Source: CAD feature listing. Evaluate the final solid. Frame: model axes, mm. A direction names the side the tool comes from. Give positions to 0.01 mm unless a question says otherwise; leave off trailing zeros. Order: outer loops, then holes, each group sorted by start corner. A loop starts at its lowest first (then second) coordinate and runs counter-clockwise, first axis right, second up.
1) Section C-C, the plane x = -3.25. Return loops of the section in (y, z).
2) Material intervals for line 1 (Y direction, x = -5, z = 7.5); line 2 (Z direction, x = 9.5, y = -14.25); line 3 (Z direction, x = 7.5, y = -14.5), sorted ascending.
3) First-contact query: P1, Ø5, axis at x = 2.5, z = 6, coming from the +Y side; P2, Ø2, axis at x = 10, z = -1.5, coming from the -Y side. Flat tips, straight axial feed; report the tip coordinate or a pass-through.
4) Access query for faces 5 (the face through (0, -12.7, -4)), 6 (the face through (-8, -17.018, -12)). Directions: +Z, -Z, +X, -X, +Y, -Y. A direction counts if a zero-diameter tool reaches every point of the face in a straight line with its end or side. Return the directions, or none.
5) Section A-A, the plane x = 8.25. Return loops of the section in (y, z).
6) Draft query along X for faces 1 (the face through (-4.62, -14.83, 5.84)), 2 (the face through (-12.639, -6, -4)), 3 (the face through (12.761, -6, -4)), 4 (the face through (0, -6, -16.45)). Return one class per face: released by +X, released by -X, zero draft, split by the parting line, or undercut.
7) Section B-B, the plane z = 6.5. Return loops of the section in (x, y).
8) Section D-D, the plane z = -6.75. Return loops of the section in (x, y), plus the area to 3 significant figures.
```python
from build123d import *

# Parameters (mm, degrees)
F0_W     = 25.4
F0_H     = 25.4
F1_DEPTH = 12.7
F2_R     = 3.892272
F3_DEPTH = 17.018
F2_R_2   = 3.825823
F4_DEPTH = 17.018
F2_R_3   = 3.864432
F5_DEPTH = 17.018
F2_R_4   = 3.786819
F6_DEPTH = 17.018


with BuildPart() as f1:
    # F0 (on Front) → F1 (new body)
    with BuildSketch(Plane.XZ):
        with Locations((0.061012, -3.750413)):
            Rectangle(F0_W, F0_H)
    extrude(amount=F1_DEPTH)

    # F2 (on Front) → F3 (join)
    with BuildSketch(Plane.XZ):
        with Locations((-8.308703, -12.045457)):
            Circle(F2_R)
    extrude(amount=F3_DEPTH)

    # F2 (on Front) → F4 (join)
    with BuildSketch(Plane.XZ):
        with Locations((8.594656, -12.16163)):
            Circle(F2_R_2)
    extrude(amount=F4_DEPTH)

    # F2 (on Front) → F5 (join)
    with BuildSketch(Plane.XZ):
        with Locations((-8.308703, 4.683642)):
            Circle(F2_R_3)
    extrude(amount=F5_DEPTH)

    # F2 (on Front) → F6 (join)
    with BuildSketch(Plane.XZ):
        with Locations((8.594656, 4.683642)):
            Circle(F2_R_4)
    extrude(amount=F6_DEPTH)


solid = f1.part
```
From the geometry:
1. outline: (-12.7, -16.45) - (0, -16.45) - (0, 8.95) - (-12.7, 8.95) - close
2. line 1: y = -12.7 to 0
2. line 2: z = -15.88 to -8.44, 1.01 to 8.36
2. line 3: z = -15.83 to -8.5, 1.06 to 8.31
3. P1: stops at y = 0
3. P2: stops at y = -12.7
4. face 5: -Y
4. face 6: +Z, -Z, +X, -X, -Y
5. outline: (-17.02, -15.97) - (-12.7, -15.97) - (-12.7, -16.45) - (0, -16.45) - (0, 8.95) - (-12.7, 8.95) - (-12.7, 8.45) - (-17.02, 8.45) - (-17.02, 0.91) - (-12.7, 0.91) - (-12.7, -8.35) - (-17.02, -8.35) - close
6. face 1: undercut
6. face 2: released by -X
6. face 3: released by +X
6. face 4: zero draft
7. outline: (-12.64, -12.7) - (-11.72, -12.7) - (-11.72, -17.02) - (-4.9, -17.02) - (-4.9, -12.7) - (5.27, -12.7) - (5.27, -17.02) - (11.92, -17.02) - (11.92, -12.7) - (12.76, -12.7) - (12.76, 0) - (-12.64, 0) - close
8. outline: (-12.64, -12.7) - (12.76, -12.7) - (12.76, 0) - (-12.64, 0) - close
8. area: 323 mm2
